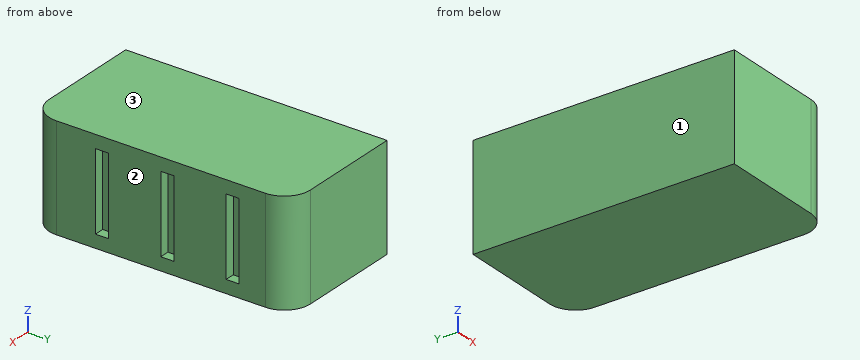
from build123d import *

# Parameters (mm, degrees)
SKETCH1_W           = 10
SKETCH1_H           = 20
BOSS_EXTRUDE1_DEPTH = 8
FILLET3_R           = 2
SKETCH2_W           = 6
SKETCH2_H           = 1
CUT_EXTRUDE1_DEPTH  = 0.75
LPATTERN1_COUNT     = 3
LPATTERN1_PITCH     = 5


with BuildPart() as part:
    # Sketch1 → Boss-Extrude1 (new body)
    with BuildSketch(Plane.XY):
        Rectangle(SKETCH1_W, SKETCH1_H)
    extrude(amount=BOSS_EXTRUDE1_DEPTH)

    # Fillet3
    fillet3_edges = [part.edges().sort_by_distance(p)[0] for p in [
        (5, 10, 4),
        (5, -10, 4),
    ]]
    fillet(fillet3_edges, radius=FILLET3_R)

    # Sketch2 → Cut-Extrude1 (cut)
    with BuildSketch(Plane(origin=(5, 0, 0), x_dir=(0, 0, -1), z_dir=(1, 0, 0))):
        with Locations((-4, -4.5)):
            Rectangle(SKETCH2_W, SKETCH2_H)
    cut_extrude1 = extrude(amount=-CUT_EXTRUDE1_DEPTH, mode=Mode.SUBTRACT)

    # LPattern1: Cut-Extrude1 ×3
    with Locations(*[(0, i * LPATTERN1_PITCH, 0) for i in range(1, LPATTERN1_COUNT)]):
        add(cut_extrude1, mode=Mode.SUBTRACT)


solid = part.part
Build history of the part. All positions in model axes, mm. Face numbers are marked on the shaded views. Round coordinates to 2 decimals unless told otherwise and drop trailing zeros. Write each loop counter-clockwise with the first axis right and the second up, starting at its lowest first coordinate (ties: lowest second). Pieces come first, ordered by that corner, then holes. Notation, with made-up numbers: (-6.5, -23.75) -> (-1.5, -23.75) arc R30 ccw to (-1.5, -0.75) -> close; hole circle Ø11 at (-14, 51.5). An arc over 180 degrees is marked (long way). Write item = value, one per line.
(1) Flat gauge pins, fed straight in: pin 1 (0.5 mm diameter, centred on y = 5.5, z = 4.5, fed in from +X); pin 2 (0.8 mm diameter, centred on x = 5, z = 2.5, fed in from +Y). Where does each tip first touch, or does it go through?
Answer:
pin_1 = 4.25
pin_2 = 9.2
(2) Two-plate mould, pull along X, no slides. Class the marked faces 1, 2 and 3: pulls with the +X half, pulls with the -X half, needs draft (parallel to the pull), parting line crosses it, or undercut.
Answer:
face_1 = pulls with the -X half
face_2 = pulls with the +X half
face_3 = needs draft
(3) Probe L1, parallel to Y at x = 4.5, z = 2; L2, parallel to X at y = 5.5, z = 6.5; L3, parallel to Y at x = 3.75, z = 3.5. List the from-to ranges inside material, lowest first.
Answer:
L1 = -9.32 to -5, -4 to 0, 1 to 5, 6 to 9.32
L2 = -5 to 4.25
L3 = -9.85 to 9.85
(4) Band-saw the part on A-A (z = 6.75). Give the cut face in (x, y), then the cut area to 3 significant figures.
Answer:
outline = (-5, -10) -> (3, -10) arc R2 ccw to (5, -8) -> (5, -5) -> (4.25, -5) -> (4.25, -4) -> (5, -4) -> (5, 0) -> (4.25, 0) -> (4.25, 1) -> (5, 1) -> (5, 5) -> (4.25, 5) -> (4.25, 6) -> (5, 6) -> (5, 8) arc R2 ccw to (3, 10) -> (-5, 10) -> close
area = 196 mm2
